Check sheet for the modelled part. Datum: model origin and axes. Units: mm. Round coordinates to 2 decimals unless told otherwise and drop trailing zeros. Write each loop counter-clockwise with the first axis right and the second up, starting at its lowest first coordinate (ties: lowest second). Pieces come first, ordered by that corner, then holes.
Item 1: Cross-section at B-B on z = 6.5. Enter the section's corners in (x, y) (3 decimals).
Item 2: Material ranges on line 1 (X direction, y = -1.25, z = 5.75); line 2 (X direction, y = -1, z = 7.25); line 3 (X direction, y = 2.75, z = 1.5), recorded low to high.
Item 3: Release check for a two-part mould opening along Y. For faces 1 (the cylindrical face through (-1.38, -1.06, 3.76)), 2 (the cylindrical face through (120.61, 0.08, 3.76)), 3 (the flat face through (60, 0, 7.62)), 4 (the flat face through (60, -4.445, 4)) record: +Y half, -Y half, draft (parallel to the pull), parting line (faces both ways), or undercut.
Item 4: Cross-section at A-A on y = 0. Enter the section's corners in (x, z) (3 decimals).
Item 5: Go/stop test with a flat-tipped pin: pin 1 Ø1 at (y, z) = (-2.5, 5) entering from +X. Record where the tip stops, or that it passes through.
from build123d import *

# Parameters (mm, degrees)
BOSS_EXTRUDE1_DEPTH = 7.62
CUT_EXTRUDE1_START  = -8.62
SKETCH2_R           = 1.7399
CUT_EXTRUDE1_DEPTH  = 9.62


with BuildPart() as part:
    # Sketch1 → Boss-Extrude1 (new body)
    with BuildSketch(Plane.XY):
        with BuildLine():
            Line((0, 4.445), (118.872, 4.445))
            ThreePointArc((118.872, 4.445), (123.317, 0), (118.872, -4.445))
            Line((118.872, -4.445), (0, -4.445))
            ThreePointArc((0, -4.445), (-4.445, 0), (0, 4.445))
        make_face()
    extrude(amount=BOSS_EXTRUDE1_DEPTH)

    # Sketch2 → Cut-Extrude1 (cut)
    with BuildSketch(Plane.XY.offset(7.62).offset(CUT_EXTRUDE1_START)):
        Circle(SKETCH2_R)
    cut_extrude1 = extrude(amount=CUT_EXTRUDE1_DEPTH, mode=Mode.SUBTRACT)

    # Mirror1: Cut-Extrude1 across plane
    add(cut_extrude1.mirror(Plane(origin=(59.436, 0, 0), x_dir=(0, 0, 1), z_dir=(1, 0, 0))), mode=Mode.SUBTRACT)


solid = part.part
Response values:
1. outline: (0, -4.445) - (118.872, -4.445) arc R4.445 ccw to (118.872, 4.445) - (0, 4.445) arc R4.445 ccw to start; hole circle Ø3.48 at (0, 0); hole circle Ø3.48 at (118.872, 0)
2. line 1: x = -4.27 to -1.21, 1.21 to 117.66, 120.08 to 123.14
2. line 2: x = -4.33 to -1.42, 1.42 to 117.45, 120.3 to 123.2
2. line 3: x = -3.49 to 122.36
3. face 1: undercut
3. face 2: undercut
3. face 3: draft
3. face 4: -Y half
4. outline: (-4.445, 0) - (-1.74, 0) - (-1.74, 7.62) - (-4.445, 7.62) - close; (1.74, 0) - (117.132, 0) - (117.132, 7.62) - (1.74, 7.62) - close; (120.612, 0) - (123.317, 0) - (123.317, 7.62) - (120.612, 7.62) - close
5. pin 1: stops at x = 122.84
